Can you work these out from the model? Positions are in its coordinate system, mm. Face numbers are marked on the shaded views. A direction names the side the tool comes from. Coordinates: 2 decimals unless noted, no trailing zeros. Loops run counter-clockwise (first coordinate to the right, second up) from the corner with the lowest first, then second, coordinate; pieces in that order, holes last.
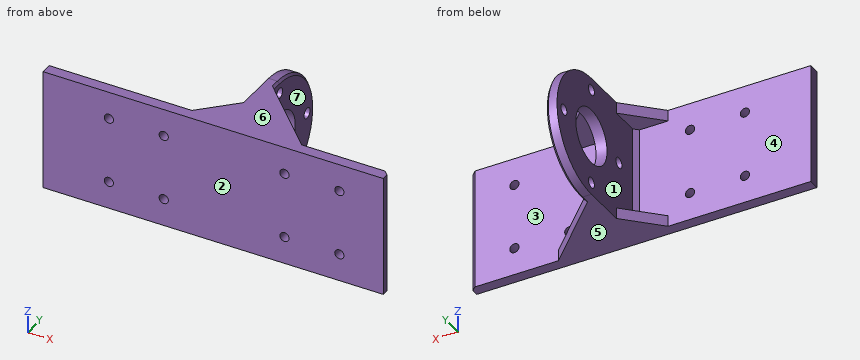
```python
from build123d import *

# Parameters (mm, degrees)
SKETCH_1_R          = 12.5
SKETCH_1_R_2        = 2.4
EXTRUDE_1_DEPTH     = 5
SKETCH_2_W          = 55
SKETCH_2_H          = 5
EXTRUDE_2_DEPTH     = 80
RIB_1_REACH         = 105.712
SKETCH_3_WALL_W     = 230.637888562
SKETCH_3_WALL_H     = 5
CHAMFER_2_SIZE      = 2
SKETCH_4_W          = 55
SKETCH_4_H          = 5
EXTRUDE_3_DEPTH     = 70
RIB_6_REACH         = 105.712
SKETCH_5_WALL_W     = 251.851091998
SKETCH_5_WALL_H     = 5
CUT_EXTRUDE_1_REACH = 107.178
SKETCH_6_R          = 2.1
CHAMFER_3_SIZE      = 1
CHAMFER_4_SIZE      = 2


with BuildPart() as part:
    # 草图1 → 凸台-拉伸1 (new body)
    with BuildSketch(Plane(origin=(0, 0, 0), x_dir=(0, 0, -1), z_dir=(1, 0, 0))):
        with BuildLine():
            Line((-27.5, 0), (-27.5, -40))
            Line((-27.5, -40), (27.5, -40))
            Line((27.5, -40), (27.5, 0))
            ThreePointArc((27.5, 0), (0, 27.5), (-27.5, 0))
        make_face()
        Circle(SKETCH_1_R, mode=Mode.SUBTRACT)
        with Locations((0, 22)):
            Circle(SKETCH_1_R_2, mode=Mode.SUBTRACT)
        with Locations((22, 0)):
            Circle(SKETCH_1_R_2, mode=Mode.SUBTRACT)
        with Locations((0, -22)):
            Circle(SKETCH_1_R_2, mode=Mode.SUBTRACT)
        with Locations((-22, 0)):
            Circle(SKETCH_1_R_2, mode=Mode.SUBTRACT)
    extrude(amount=EXTRUDE_1_DEPTH)

    # 草图2 → 凸台-拉伸2 (add)
    with BuildSketch(Plane.ZY):
        with Locations((0, -37.5)):
            Rectangle(SKETCH_2_W, SKETCH_2_H)
    extrude(amount=EXTRUDE_2_DEPTH)

    # 草图3 wall → 筋1 (add, up to next)
    with BuildSketch(Plane(origin=(-7.5, -27.5, 25), x_dir=(0.707106781187, 0.707106781187, 0), z_dir=(-0.707106781187, 0.707106781187, 0)), mode=Mode.PRIVATE) as rib_1_sk1:
        Rectangle(SKETCH_3_WALL_W, SKETCH_3_WALL_H)
    rib_1_tool1 = extrude(rib_1_sk1.sketch, amount=-RIB_1_REACH, mode=Mode.PRIVATE) - part.part
    rib_1 = rib_1_tool1.solids().sort_by_distance((-7.5, -27.5, 25))[0]
    add(rib_1)

    # 镜向1: 筋1 across plane
    add(rib_1.mirror(Plane.XY))

    # 倒角2
    chamfer_2_edges = [part.edges().sort_by_distance(p)[0] for p in [
        (0, -35, 0),
    ]]
    chamfer(chamfer_2_edges, length=CHAMFER_2_SIZE)

    # 草图4 → 凸台-拉伸3 (add)
    with BuildSketch(Plane(origin=(5, 0, 0), x_dir=(0, 0, -1), z_dir=(1, 0, 0))):
        with Locations((0, -37.5)):
            Rectangle(SKETCH_4_W, SKETCH_4_H)
    extrude(amount=EXTRUDE_3_DEPTH)

    # 草图5 wall → 筋6 (add, up to next)
    with BuildSketch(Plane(origin=(20, -20, 25), x_dir=(-0.707106781187, 0.707106781187, 0), z_dir=(-0.707106781187, -0.707106781187, 0)), mode=Mode.PRIVATE) as rib_6_sk1:
        Rectangle(SKETCH_5_WALL_W, SKETCH_5_WALL_H)
    rib_6_tool1 = extrude(rib_6_sk1.sketch, amount=RIB_6_REACH, mode=Mode.PRIVATE) - part.part
    rib_6 = rib_6_tool1.solids().sort_by_distance((20, -20, 25))[0]
    add(rib_6)

    # 镜向2: 筋6 across plane
    add(rib_6.mirror(Plane.XY))

    # 草图6 → 切除-拉伸1 (cut, up to next)
    with BuildSketch(Plane(origin=(0, -35, 0), x_dir=(1, 0, 0), z_dir=(0, 1, 0)), mode=Mode.PRIVATE) as cut_extrude_1_sk1:
        with Locations(Location((30, 15, 0), (0, 0, 270))):
            Circle(SKETCH_6_R)
    cut_extrude_1_tool1 = extrude(cut_extrude_1_sk1.sketch, amount=-CUT_EXTRUDE_1_REACH, mode=Mode.PRIVATE) & part.part
    # 草图6 → 切除-拉伸1 (cut, up to next)
    with BuildSketch(Plane(origin=(0, -35, 0), x_dir=(1, 0, 0), z_dir=(0, 1, 0)), mode=Mode.PRIVATE) as cut_extrude_1_sk2:
        with Locations(Location((55, 15, 0), (0, 0, 270))):
            Circle(SKETCH_6_R)
    cut_extrude_1_tool2 = extrude(cut_extrude_1_sk2.sketch, amount=-CUT_EXTRUDE_1_REACH, mode=Mode.PRIVATE) & part.part
    # 草图6 → 切除-拉伸1 (cut, up to next)
    with BuildSketch(Plane(origin=(0, -35, 0), x_dir=(1, 0, 0), z_dir=(0, 1, 0)), mode=Mode.PRIVATE) as cut_extrude_1_sk3:
        with Locations(Location((-50, 15, 0), (0, 0, 270))):
            Circle(SKETCH_6_R)
    cut_extrude_1_tool3 = extrude(cut_extrude_1_sk3.sketch, amount=-CUT_EXTRUDE_1_REACH, mode=Mode.PRIVATE) & part.part
    # 草图6 → 切除-拉伸1 (cut, up to next)
    with BuildSketch(Plane(origin=(0, -35, 0), x_dir=(1, 0, 0), z_dir=(0, 1, 0)), mode=Mode.PRIVATE) as cut_extrude_1_sk4:
        with Locations(Location((-25, 15, 0), (0, 0, 270))):
            Circle(SKETCH_6_R)
    cut_extrude_1_tool4 = extrude(cut_extrude_1_sk4.sketch, amount=-CUT_EXTRUDE_1_REACH, mode=Mode.PRIVATE) & part.part
    # 草图6 → 切除-拉伸1 (cut, up to next)
    with BuildSketch(Plane(origin=(0, -35, 0), x_dir=(1, 0, 0), z_dir=(0, 1, 0)), mode=Mode.PRIVATE) as cut_extrude_1_sk5:
        with Locations(Location((55, -15, 0), (0, 0, 270))):
            Circle(SKETCH_6_R)
    cut_extrude_1_tool5 = extrude(cut_extrude_1_sk5.sketch, amount=-CUT_EXTRUDE_1_REACH, mode=Mode.PRIVATE) & part.part
    # 草图6 → 切除-拉伸1 (cut, up to next)
    with BuildSketch(Plane(origin=(0, -35, 0), x_dir=(1, 0, 0), z_dir=(0, 1, 0)), mode=Mode.PRIVATE) as cut_extrude_1_sk6:
        with Locations(Location((30, -15, 0), (0, 0, 270))):
            Circle(SKETCH_6_R)
    cut_extrude_1_tool6 = extrude(cut_extrude_1_sk6.sketch, amount=-CUT_EXTRUDE_1_REACH, mode=Mode.PRIVATE) & part.part
    # 草图6 → 切除-拉伸1 (cut, up to next)
    with BuildSketch(Plane(origin=(0, -35, 0), x_dir=(1, 0, 0), z_dir=(0, 1, 0)), mode=Mode.PRIVATE) as cut_extrude_1_sk7:
        with Locations(Location((-25, -15, 0), (0, 0, 270))):
            Circle(SKETCH_6_R)
    cut_extrude_1_tool7 = extrude(cut_extrude_1_sk7.sketch, amount=-CUT_EXTRUDE_1_REACH, mode=Mode.PRIVATE) & part.part
    # 草图6 → 切除-拉伸1 (cut, up to next)
    with BuildSketch(Plane(origin=(0, -35, 0), x_dir=(1, 0, 0), z_dir=(0, 1, 0)), mode=Mode.PRIVATE) as cut_extrude_1_sk8:
        with Locations(Location((-50, -15, 0), (0, 0, 270))):
            Circle(SKETCH_6_R)
    cut_extrude_1_tool8 = extrude(cut_extrude_1_sk8.sketch, amount=-CUT_EXTRUDE_1_REACH, mode=Mode.PRIVATE) & part.part
    add(cut_extrude_1_tool1.solids().sort_by_distance((30, -35, -15))[0], mode=Mode.SUBTRACT)
    add(cut_extrude_1_tool2.solids().sort_by_distance((55, -35, -15))[0], mode=Mode.SUBTRACT)
    add(cut_extrude_1_tool3.solids().sort_by_distance((-50, -35, -15))[0], mode=Mode.SUBTRACT)
    add(cut_extrude_1_tool4.solids().sort_by_distance((-25, -35, -15))[0], mode=Mode.SUBTRACT)
    add(cut_extrude_1_tool5.solids().sort_by_distance((55, -35, 15))[0], mode=Mode.SUBTRACT)
    add(cut_extrude_1_tool6.solids().sort_by_distance((30, -35, 15))[0], mode=Mode.SUBTRACT)
    add(cut_extrude_1_tool7.solids().sort_by_distance((-25, -35, 15))[0], mode=Mode.SUBTRACT)
    add(cut_extrude_1_tool8.solids().sort_by_distance((-50, -35, 15))[0], mode=Mode.SUBTRACT)

    # 倒角3
    chamfer_3_edges = [part.edges().sort_by_distance(p)[0] for p in [
        (5, -2.5, -27.5),
        (5, 27.5, 0),
        (5, -2.5, 27.5),
    ]]
    chamfer(chamfer_3_edges, length=CHAMFER_3_SIZE)

    # 倒角4
    chamfer_4_edges = [part.edges().sort_by_distance(p)[0] for p in [
        (75, -35, 0),
    ]]
    chamfer(chamfer_4_edges, length=CHAMFER_4_SIZE)


solid = part.part
```
(1) I want a section at A-A on x = -50. Write out the boundary of the cut face in (y, z).
Check values:
outline: (-40, -27.5) - (-35, -27.5) - (-35, -17.1) - (-40, -17.1) - close; (-40, -12.9) - (-35, -12.9) - (-35, 12.9) - (-40, 12.9) - close; (-40, 17.1) - (-35, 17.1) - (-35, 27.5) - (-40, 27.5) - close
(2) If we mould it in two halves opening along Z, with no side actions, what happens to the marked faces 4, 5, 6 and 7? For each: released by +Z, released by -Z, zero draft, split by the parting line, or undercut.
Check values:
face 4: undercut
face 5: released by -Z
face 6: released by +Z
face 7: undercut
(3) I want a section at B-B on z = 0. Write out the boundary of the cut face in (x, y), then the cut area to 3 significant figures.
Check values:
outline: (-80, -40) - (75, -40) - (75, -37) - (73, -35) - (5, -35) - (5, -24.4) - (0, -24.4) - (0, -33) - (-2, -35) - (-80, -35) - close; (0, -19.6) - (5, -19.6) - (5, -12.5) - (0, -12.5) - close; (0, 12.5) - (5, 12.5) - (5, 19.6) - (0, 19.6) - close; (0, 24.4) - (5, 24.4) - (5, 26.5) - (4, 27.5) - (0, 27.5) - close
area: 914 mm2
(4) I want a section at D-D on x = 10. Write out the boundary of the cut face in (y, z), then the cut area to 3 significant figures.
Check values:
outline: (-40, -27.5) - (-10, -27.5) - (-10, -22.5) - (-35, -22.5) - (-35, 22.5) - (-10, 22.5) - (-10, 27.5) - (-40, 27.5) - close
area: 525 mm2
(5) I'm going to push flat-ended pins straight in: pin 1 (3 mm diameter, centred on y = -23.5, z = -12.5, fed in from +X); pin 2 (4.5 mm diameter, centred on y = -22, z = 0, fed in from +X); pin 3 (5.5 mm diameter, centred on x = -25, z = -15, fed in from +Y); pin 4 (1.5 mm diameter, centred on y = -16, z = -3, fed in from -X). Where does each tip first touch, or does it pass through?
Check values:
pin 1: stops at x = 5
pin 2: passes through
pin 3: stops at y = -35
pin 4: stops at x = 0
(6) I want a section at C-C on y = -22. Write out the boundary of the cut face in (x, z), then the cut area to 3 significant figures.
Check values:
outline: (-2, -27.5) - (22, -27.5) - (22, -22.5) - (5, -22.5) - (5, -2.4) - (0, -2.4) - (0, -22.5) - (-2, -22.5) - close; (-2, 22.5) - (0, 22.5) - (0, 2.4) - (5, 2.4) - (5, 22.5) - (22, 22.5) - (22, 27.5) - (-2, 27.5) - close
area: 441 mm2
(7) If I drill on probe 1 along X at (y, z) = (-38.3, 15); probe 2 along Y at (x, z) = (3, 0); probe 3 along X at (y, z) = (-36, -15), over which ranges is the centre line in solid material (lowest first)?
Check values:
probe 1: x = -80 to -52.1, -47.9 to -27.1, -22.9 to 27.9, 32.1 to 52.9, 57.1 to 75
probe 2: y = -40 to -24.4, -19.6 to -12.5, 12.5 to 19.6, 24.4 to 27.5
probe 3: x = -80 to -52.1, -47.9 to -27.1, -22.9 to 27.9, 32.1 to 52.9, 57.1 to 74
(8) Which directions (+Z, -Z, +X, -X, +Y, -Y) give clear straight access to the entire face, cutting with the end or side of a thin tool? Please do the marked faces 1, 2 and 3.
Check values:
face 1: -X, +Y
face 2: +Z, -Z, +X, -X, -Y
face 3: +X, +Y
